```python
from build123d import *

# Parameters (mm, degrees)
BOSS_EXTRU_1_DEPTH = 1.3


with BuildPart() as part:
    # Esquisse1 → Révolution1 (revolve)
    with BuildSketch(Plane.XY, mode=Mode.PRIVATE) as r_volution1_sk:
        with BuildLine():
            Line((0, 2), (0, -12.5))
            Line((0, -12.5), (1.5, -12.5))
            Line((1.5, -12.5), (1.5, -4.5))
            Line((1.5, -4.5), (2.75, -4.5))
            Line((2.75, -4.5), (2.75, -3.2))
            Line((2.75, -3.2), (1.25, -3.2))
            Line((1.25, -3.2), (1.25, -1.5612495))
            ThreePointArc((1.25, -1.5612495), (1.887127314, 0.662382443), (0, 2))
        make_face()
    revolve(r_volution1_sk.sketch.rotate(Axis((0, 0, 0), (0, 1, 0)), 90), axis=Axis((0, 0, 0), (0, 1, 0)))

    # Esquisse2 → Boss.-Extru.1 (add)
    with BuildSketch(Plane(origin=(0, -3.2, 0), x_dir=(1, 0, 0), z_dir=(0, 1, 0))):
        Polygon((1.58771324, 2.75), (-1.58771324, 2.75), (-3.175426481, 0), (-1.58771324, -2.75), (1.58771324, -2.75), (3.175426481, 0), align=None)
    extrude(amount=-BOSS_EXTRU_1_DEPTH)


solid = part.part
```
Work out the finished part from the listing and answer in its coordinate system (mm). A direction names the side the tool comes from. Give positions to 0.01 mm unless a question says otherwise; leave off trailing zeros. Loops run counter-clockwise (first coordinate to the right, second up) from the corner with the lowest first, then second, coordinate; pieces in that order, holes last. Notation, with made-up numbers: (66.25, -36.5) -> (104.25, -36.5) arc R21 cw to (104.25, -24.5) -> close; hole circle Ø7 at (-14.75, -17.5). An arc over 180 degrees is marked (long way). Put each result on its own line as item: value. Start each with the question number.
Item 1: The part is cut by section B-B (x = -1.75). Give the vertices of the cut face in (y, z).
Item 2: The part is cut by section C-C (y = -7.5). Give the vertices of the cut face in (x, z).
Item 3: The part is cut by section D-D (z = -0.2). Give the vertices of the cut face in (x, y).
Item 4: The mould has two halves that part along Y. Classify faces 1 (the face through (-2.37, -3.841, -1.394)), 2 (the face through (1, -3.2, -1)), 3 (the face through (0, -12.5, 0)): released by +Y, released by -Y, zero draft, split by the parting line, or undercut.
Item 5: Which of the six approach directions +Z, -Z, +X, -X, +Y, -Y give full straight-line access (tool end or side, diameter ignored) to faces 4 (the face through (-0.05, -2.37, 1.25)), 5 (the face through (1.4, -4.5, -1.3)), 6 (the face through (2.37, -3.841, 1.394))?
Item 6: The part is cut by section A-A (x = 0). Give the vertices of the cut face in (y, z).
Item 7: Find the intervals of material crossed by L1, parallel to Y at x = -1, z = 1.85; L2, parallel to Y at x = 0.5, z = -1.55; L3, parallel to X at y = -12, z = 0.45, in increasing order. Write a range as [from, to].
Item 8: Each of these flat-tipped pins is pushed along its axis until it touches: P1, Ø2, axis at x = -2, z = 1.5, coming from the +Y side; P2, Ø1, axis at y = -3, z = 1.5, coming from the +X side. Where does it stop, or does it pass through?
Answers below:
1. outline: (-4.5, -2.47) -> (-3.2, -2.47) -> (-3.2, 2.47) -> (-4.5, 2.47) -> close; circle Ø1.94 at (0, 0)
2. outline: circle Ø3 at (0, 0)
3. outline: (-3.06, -4.5) -> (-1.49, -4.5) -> (-1.49, -12.5) -> (1.49, -12.5) -> (1.49, -4.5) -> (3.06, -4.5) -> (3.06, -3.2) -> (1.23, -3.2) -> (1.23, -1.56) arc R1.99 ccw (long way) to (-1.23, -1.56) -> (-1.23, -3.2) -> (-3.06, -3.2) -> close
4. face 1: zero draft
4. face 2: undercut
4. face 3: released by -Y
5. face 4: none
5. face 5: -Y
5. face 6: +Z, +X, +Y, -Y
6. outline: (-12.5, -1.5) -> (-4.5, -1.5) -> (-4.5, -2.75) -> (-3.2, -2.75) -> (-3.2, -1.25) -> (-1.56, -1.25) arc R2 ccw (long way) to (-1.56, 1.25) -> (-3.2, 1.25) -> (-3.2, 2.75) -> (-4.5, 2.75) -> (-4.5, 1.5) -> (-12.5, 1.5) -> close
7. L1: [-4.5, -3.2]
7. L2: [-4.5, -3.2], [-1.16, 1.16]
7. L3: [-1.43, 1.43]
8. P1: y = 1.32
8. P2: x = 2.57
